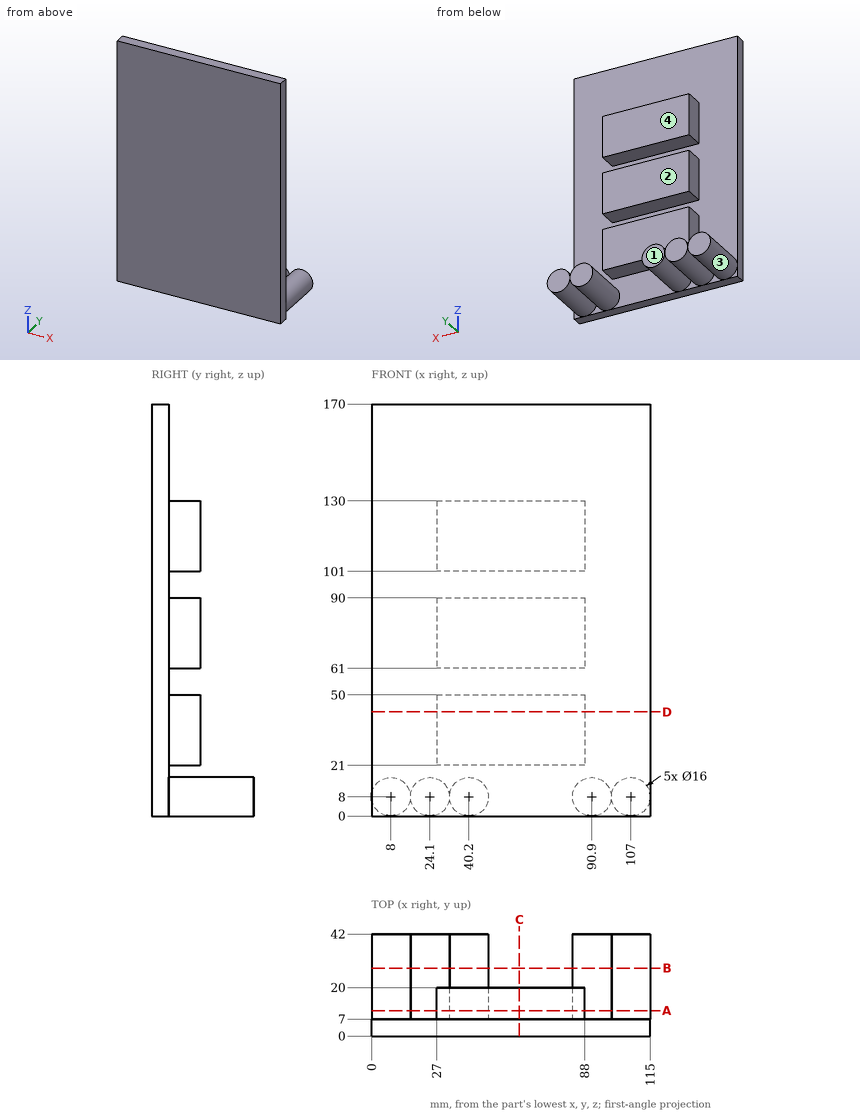
Here's the drawing with two shaded views (mm, measured from the low corner). I have some questions. A direction names the side the tool comes from. Give positions to 0.01 mm unless a question says otherwise; leave off trailing zeros. Loops run counter-clockwise (first coordinate to the right, second up) from the corner with the lowest first, then second, coordinate; pieces in that order, holes last. Notation, with made-up numbers: (44.5, 89.5) -> (77.5, 89.5) arc R21 cw to (77.5, 95.5) -> close; hole circle Ø1 at (32.25, 61.5). An arc over 180 degrees is marked (long way). Answer as a JSON object with one key per item and string values. Group by question number.
Item 1: Imagine slicing it at D-D on z = 43. Write out the boundary of the cut face in (x, y), then the cut area to 3 significant figures.
Item 2: Imagine slicing it at C-C on x = 61. Write out the boundary of the cut face in (y, z).
Item 3: On a 3-axis mill with a long thin cutter (end or side, diameter ignored), from which of +Z, -Z, +X, -X, +Y, -Y can I reach the whole of each face in a straight line? I mean the marked faces 1 and 2. Say none if no direction works.
Item 4: Thinking about a two-plate mould opening in X: for the marked faces 3 and 4, which applies, pulls with the +X half, pulls with the -X half, needs draft (parallel to the pull), parting line crosses it, or undercut?
Item 5: Imagine slicing it at B-B on y = 28. Write out the boundary of the cut face in (x, z).
Item 6: Imagine slicing it at A-A on y = 10.5. Write out the boundary of the cut face in (x, z), then the cut area to 3 significant figures.
Item 7: I need wall thicknesses on L1, parallel to Z at x = 62.5, y = 13.5; L2, parallel to Z at x = 37.5, y = 9; L3, parallel to Z at x = 30, y = 9. Which ranges of each line are inside material? Lowest first, please.
Item 8: Will these pins go through, and if not, where does the flat tip stop? pin 1 (8 mm diameter, centred on y = 23.5, z = 25, fed in from +X); pin 2 (23 mm diameter, centred on x = 72.5, z = 118, fed in from +Y); pin 3 (6.5 mm diameter, centred on y = 14, z = 75.5, fed in from -X).
Answer list:
{
 "1": {"outline": "(0, 0) -> (115, 0) -> (115, 7) -> (88, 7) -> (88, 20) -> (27, 20) -> (27, 7) -> (0, 7) -> close", "area": "1,600 mm2"},
 "2": {"outline": "(0, 0) -> (7, 0) -> (7, 21) -> (20, 21) -> (20, 50) -> (7, 50) -> (7, 61) -> (20, 61) -> (20, 90) -> (7, 90) -> (7, 101) -> (20, 101) -> (20, 130) -> (7, 130) -> (7, 170) -> (0, 170) -> close"},
 "3": {"face 1": "+Z, -Z, +X, -X, +Y", "face 2": "+Z, +X, -X, +Y"},
 "4": {"face 3": "undercut", "face 4": "needs draft"},
 "5": {"outline": "circle Ø16 at (8, 8); circle Ø16 at (24.1, 8); circle Ø16 at (40.2, 8); circle Ø16 at (90.9, 8); circle Ø16 at (107, 8)"},
 "6": {"outline": "circle Ø16 at (8, 8); circle Ø16 at (24.1, 8); (27, 21) -> (88, 21) -> (88, 50) -> (27, 50) -> close; (27, 61) -> (88, 61) -> (88, 90) -> (27, 90) -> close; (27, 101) -> (88, 101) -> (88, 130) -> (27, 130) -> close; circle Ø16 at (40.2, 8); circle Ø16 at (90.9, 8); circle Ø16 at (107, 8)", "area": "6,310 mm2"},
 "7": {"L1": "z = 21 to 50, 61 to 90, 101 to 130", "L2": "z = 0.47 to 15.53, 21 to 50, 61 to 90, 101 to 130", "L3": "z = 2.6 to 13.4, 21 to 50, 61 to 90, 101 to 130"},
 "8": {"pin 1": "stops at x = 88", "pin 2": "stops at y = 20", "pin 3": "stops at x = 27"}
}
